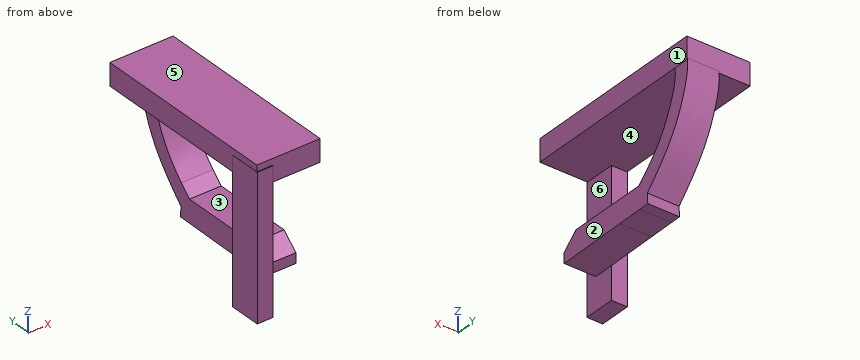
from build123d import *

# Parameters (mm, degrees)
F0_W          = 12.7
F0_H          = 57.15
F1_DEPTH      = 6.35
F3_W          = 25.4
F3_H          = 76.2
F4_DEPTH      = 6.35
F4_DEPTH_BACK = 2.54
F7_DEPTH      = 12.7


with BuildPart() as f1:
    # F0 (on Right) → F1 (new body)
    with BuildSketch(Plane.YZ):
        Rectangle(F0_W, F0_H)
    extrude(amount=-F1_DEPTH)

    # F3 (on offset) → F4 (join, two sides)
    with BuildSketch(Plane.XY.offset(28.575)) as f4_sk:
        with Locations((6.4234920739, 32.0478732836)):
            Rectangle(F3_W, F3_H)
    extrude(amount=-F4_DEPTH)
    extrude(f4_sk.sketch, amount=F4_DEPTH_BACK)

    # F6 (on offset) → F7 (join)
    with BuildSketch(Plane.YZ.offset(6.35)):
        with BuildLine():
            add(Edge.make_bspline(
                [(70.2633336186, 22.8392183781), (70.4233882553, 21.3594202626), (70.8861297069, 17.0811066655), (64.7810650809, -1.7378247981), (54.8334581019, -12.2566322998), (49.6061965824, -17.6021996762)],
                knots=[0, 0, 0, 0, 0.1426234456, 0.4123453195, 0.7089617498, 0.7089617498, 0.7089617498, 0.7089617498], degree=3))
            Line((70.2633336186, 22.8392183781), (63.8625249267, 22.2573280334))
            add(Edge.make_bspline(
                [(63.8625249267, 22.2573280334), (64.0412796019, 20.8723429335), (64.5683260106, 16.7888054132), (58.9062733043, 1.7794154409), (51.9438558064, -6.0723920348), (49.3872103067, -8.6279157552)],
                knots=[0, 0, 0, 0, 0.1493923045, 0.440473389, 0.6031634486, 0.6031634486, 0.6031634486, 0.6031634486], degree=3))
            add(Edge.make_bspline(
                [(49.3872103067, -8.6279157552), (47.9749044151, -10.0396019693), (46.5441619109, -11.3720779909), (45.1433620447, -12.6561271027)],
                knots=[0.6031634486, 0.6031634486, 0.6031634486, 0.6031634486, 0.6930343867, 0.6930343867, 0.6930343867, 0.6930343867], degree=3))
            add(Edge.make_bspline(
                [(45.1433620447, -12.6561271027), (44.389197075, -13.3474356064), (42.4890896803, -15.0736774227), (40.6944116755, -16.7399375724), (39.6315032844, -17.7367295919)],
                knots=[0.6930343867, 0.6930343867, 0.6930343867, 0.6930343867, 0.7414192524, 0.8163585632, 0.8163585632, 0.8163585632, 0.8163585632], degree=3))
            Line((39.6315032844, -17.7367295919), (49.6061965824, -17.6021996762))
        make_face()
        with BuildLine():
            Line((49.8050153623, -21.68060241), (49.6061965824, -17.6021996762))
            add(Edge.make_bspline(
                [(49.6061965824, -17.6021996762), (48.2481731115, -18.9909585771), (46.8889847211, -20.3686756001), (45.5289398536, -21.7382743664)],
                knots=[0.7089617498, 0.7089617498, 0.7089617498, 0.7089617498, 0.7860216162, 0.7860216162, 0.7860216162, 0.7860216162], degree=3))
            Line((45.5289398536, -21.7382743664), (49.8050153623, -21.68060241))
        make_face()
        with BuildLine():
            add(Edge.make_bspline(
                [(49.6061965824, -17.6021996762), (48.2481731115, -18.9909585771), (46.8889847211, -20.3686756001), (45.5289398536, -21.7382743664)],
                knots=[0.7089617498, 0.7089617498, 0.7089617498, 0.7089617498, 0.7860216162, 0.7860216162, 0.7860216162, 0.7860216162], degree=3))
            Line((49.6061965824, -17.6021996762), (39.6315032844, -17.7367295919))
            add(Edge.make_bspline(
                [(39.6315032844, -17.7367295919), (38.1330562509, -19.1419683285), (36.6895570101, -20.5159457613), (35.2693948102, -21.8766461126)],
                knots=[0.8163585632, 0.8163585632, 0.8163585632, 0.8163585632, 0.9220050976, 0.9220050976, 0.9220050976, 0.9220050976], degree=3))
            Line((35.2693948102, -21.8766461126), (45.5289398536, -21.7382743664))
        make_face()
        with BuildLine():
            Line((6.4619160257, -18.1840918958), (39.6315032844, -17.7367295919))
            add(Edge.make_bspline(
                [(45.1433620447, -12.6561271027), (44.389197075, -13.3474356064), (42.4890896803, -15.0736774227), (40.6944116755, -16.7399375724), (39.6315032844, -17.7367295919)],
                knots=[0.6930343867, 0.6930343867, 0.6930343867, 0.6930343867, 0.7414192524, 0.8163585632, 0.8163585632, 0.8163585632, 0.8163585632], degree=3))
            Line((45.1433620447, -12.6561271027), (12.5717725605, -12.6561271027))
            Line((12.5717725605, -12.6561271027), (6.4619160257, -18.1840918958))
        make_face()
        with BuildLine():
            add(Edge.make_bspline(
                [(39.6315032844, -17.7367295919), (38.1330562509, -19.1419683285), (36.6895570101, -20.5159457613), (35.2693948102, -21.8766461126)],
                knots=[0.8163585632, 0.8163585632, 0.8163585632, 0.8163585632, 0.9220050976, 0.9220050976, 0.9220050976, 0.9220050976], degree=3))
            Line((39.6315032844, -17.7367295919), (6.4619160257, -18.1840918958))
            Line((6.4619160257, -18.1840918958), (6.5169481003, -22.2644338986))
            Line((6.5169481003, -22.2644338986), (35.2693948102, -21.8766461126))
        make_face()
    extrude(amount=F7_DEPTH)


solid = f1.part
Geometry check sheet. Reference: the model listing, model coordinates, mm. Face numbers are marked on the shaded views. A direction names the side the tool comes from. Coordinates: 2 decimals unless noted, no trailing zeros. Order: outer loops, then holes, each group sorted by start corner. A loop starts at its lowest first (then second) coordinate and runs counter-clockwise, first axis right, second up. Notation, with made-up numbers: (25, -18.5) -> (66, -18.5) arc R15 cw to (66, -12.5) -> close; hole circle Ø9 at (41.5, 25.25). An arc over 180 degrees is marked (long way). Use a Markdown table: item, result. Add a question column.
1. Cross-section at B-B (x = -5). Enter the section's corners in (y, z) (3 decimals), and give its area (3 significant figures).
2. Cross-section at C-C (z = -24). Enter the section's corners in (x, y).
3. Go/stop test with flat-tipped pins: pin 1 Ø2 at (x, y) = (14.5, 24.5) entering from -Z; pin 2 Ø22.5 at (y, z) = (30.5, -5.5) entering from -X; pin 3 Ø6 at (x, z) = (13, 21.5) entering from -Y; pin 4 Ø3 at (y, z) = (54.5, -16.5) entering from -X. Record where each tip stops, or that it passes through.
4. Mould release check, pull along Z, two halves, no side actions. Record for the marked faces 4, 5 and 6: pulls with the +Z half, pulls with the -Z half, needs draft (parallel to the pull), parting line crosses it, or undercut.
5. Material ranges on L1, parallel to X at y = 46.5, z = -20; L2, parallel to Y at x = -4.25, z = 11; L3, parallel to X at y = 1, z = -23.5, recorded low to high.
6. Cross-section at D-D (x = 2.5). Enter the section's corners in (y, z) (3 decimals), and give its area (3 significant figures).
7. Set-up check for the marked faces 1, 2 and 3: record each of +Z, -Z, +X, -X, +Y, -Y from which the full face is reachable in a straight line by a thin tool's end or side.
Filled sheet:
| question | item | result |
|---|---|---|
| 1 | outline | (-6.35, -28.575) -> (6.35, -28.575) -> (6.35, 22.225) -> (70.148, 22.225) -> (70.148, 31.115) -> (-6.052, 31.115) -> (-6.052, 28.575) -> (-6.35, 28.575) -> close |
| 1 | area | 1,320 mm2 |
| 2 | outline | (-6.35, -6.35) -> (0, -6.35) -> (0, 6.35) -> (-6.35, 6.35) -> close |
| 3 | pin 1 | z = -22.04 |
| 3 | pin 2 | x = 6.35 |
| 3 | pin 3 | y = -6.05 |
| 3 | pin 4 | through |
| 4 | face 4 | undercut |
| 4 | face 5 | pulls with the +Z half |
| 4 | face 6 | needs draft |
| 5 | L1 | 6.35 to 19.05 |
| 5 | L2 | -6.35 to 6.35 |
| 5 | L3 | -6.35 to 0 |
| 6 | outline | (-6.052, 22.225) -> (70.148, 22.225) -> (70.148, 31.115) -> (-6.052, 31.115) -> close |
| 6 | area | 677 mm2 |
| 7 | face 1 | +Z, -Z, +X, +Y, -Y |
| 7 | face 2 | -Z, +X, +Y, -Y |
| 7 | face 3 | +X, -X, -Y |
